from build123d import *

# Parameters (mm, degrees)
ESBO_O1_R                = 15
RESSALTO_EXTRUS_O1_DEPTH = 10
ESBO_O2_R                = 6
RESSALTO_EXTRUS_O2_DEPTH = 35
ESBO_O3_R                = 4
RESSALTO_EXTRUS_O3_DEPTH = 10
CHANFRO1_SIZE            = 2


with BuildPart() as part:
    # Esboço1 → Ressalto-extrusão1 (new body)
    with BuildSketch(Plane.XY):
        Circle(ESBO_O1_R)
    extrude(amount=RESSALTO_EXTRUS_O1_DEPTH)

    # Esboço2 → Ressalto-extrusão2 (add)
    with BuildSketch(Plane.XY.offset(10)):
        Circle(ESBO_O2_R)
    extrude(amount=RESSALTO_EXTRUS_O2_DEPTH)

    # Esboço3 → Ressalto-extrusão3 (add)
    with BuildSketch(Plane.XY.offset(45)):
        Circle(ESBO_O3_R)
    extrude(amount=RESSALTO_EXTRUS_O3_DEPTH)

    # Chanfro1
    chanfro1_edges = [part.edges().sort_by_distance(p)[0] for p in [
        (-15, 0, 0),
    ]]
    chamfer(chanfro1_edges, length=CHANFRO1_SIZE)


solid = part.part
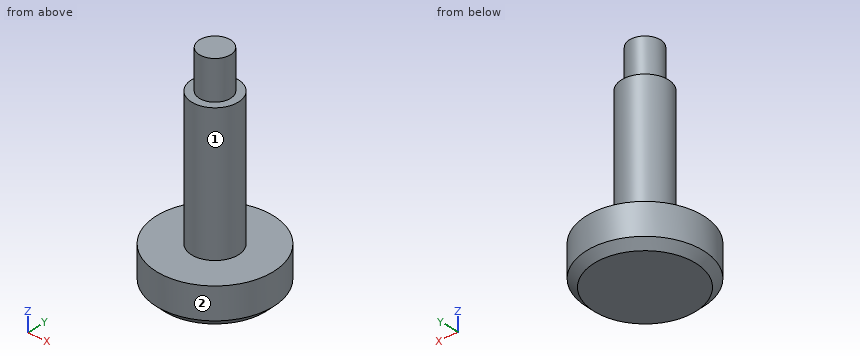
Source: CAD feature listing. Evaluate the final solid. Frame: model axes, mm. Face numbers are marked on the shaded views. A direction names the side the tool comes from. Give positions to 0.01 mm unless a question says otherwise; leave off trailing zeros. Write each loop counter-clockwise with the first axis right and the second up, starting at its lowest first coordinate (ties: lowest second). Pieces come first, ordered by that corner, then holes. Notation, with made-up numbers: M 76,-23.5 L 100,-23.5 A32 ccw 100,4.5 Z; hole C 89,15 d4. An arc over 180 degrees is marked long. Answer as a JSON object with one key per item and string values.
Q1. Contact query for flat-ended pins moving along their axis: P1, Ø1, axis at x = -3, z = 42, coming from the -Y side; P2, Ø8, axis at y = -4, z = 43, coming from the -X side; P3, Ø8, axis at y = 6, z = 32.5, coming from the -X side. Output: stop coordinate, or through.
Geometry check:
{"P1": "stops at y = -5.45", "P2": "stops at x = -6", "P3": "stops at x = -5.66"}
Q2. Cut plane D-D, the plane z = 13.5. Return the cut outline in (x, y).
Geometry check:
{"outline": "C 0,0 d12"}
Q3. Cut plane C-C, the plane z = 46. Return the cut outline in (x, y), then the cut area to 3 significant figures.
Geometry check:
{"outline": "C 0,0 d8", "area": "50.3 mm^2"}
Q4. Access query for the marked faces 1 and 2. Directions: +Z, -Z, +X, -X, +Y, -Y. A direction counts if a zero-diameter tool reaches every point of the face in a straight line with its end or side. Return the directions, or none.
Geometry check:
{"face 1": "+Z", "face 2": "+Z, -Z"}
Q5. Cut plane A-A, the plane y = 0. Return the cut outline in (x, z), then the cut area to 3 significant figures.
Geometry check:
{"outline": "M -15,2 L -13,0 L 13,0 L 15,2 L 15,10 L 6,10 L 6,45 L 4,45 L 4,55 L -4,55 L -4,45 L -6,45 L -6,10 L -15,10 Z", "area": "796 mm^2"}
Q6. Ray query, line 1 along Z through (x, y) = (8.25, -4.5); line 2 along Z through (x, y) = (2.25, 5.25); line 3 along Y through (x, z) = (-7.5, 3.5). Return the intervals inside material, ascending.
Geometry check:
{"line 1": "z = 0 to 10", "line 2": "z = 0 to 45", "line 3": "y = -12.99 to 12.99"}
